Here's how the part is built. I have some questions about the finished solid (model axes, mm). A direction names the side the tool comes from. Coordinates: 2 decimals unless noted, no trailing zeros. Loops run counter-clockwise (first coordinate to the right, second up) from the corner with the lowest first, then second, coordinate; pieces in that order, holes last. Notation, with made-up numbers: (74.25, 62) -> (107.25, 62) arc R29 ccw to (107.25, 86) -> close; hole circle Ø1 at (-38.5, 3.25). An arc over 180 degrees is marked (long way). Answer as a JSON object with one key per item and string values. Group by question number.
Q1. I want a section at B-B on y = -5. Write out the boundary of the cut face in (x, z).
Q2. I need wall thicknesses on line 1 (Z direction, x = -19, y = -0.5); line 2 (X direction, y = -6.5, z = -31); line 3 (Z direction, x = -10, y = -2.5). Which ranges of each line are inside material? Lowest first, please.
Q3. Thinking about a two-plate mould opening in Z: for faces 1 (the flat face through (6, -3, -34.366)), 2 (the flat face through (0, -4, 29.286)), 3 (the flat face through (15, -7.62, -31)), which applies, released by +Z, released by -Z, zero draft, split by the parting line, or undercut?
Q4. I want a section at A-A on z = 6.5. Write out the boundary of the cut face in (x, y), then the cut area to 3 significant figures.
Q5. I want a section at D-D on x = 18. Write out the boundary of the cut face in (y, z), then the cut area to 3 significant figures.
Q6. I'm going to push flat-ended pins straight in: pin 1 (3 mm diameter, centred on x = -17.5, z = -5.5, fed in from -Y); pin 2 (3 mm diameter, centred on x = 2.5, z = 22.5, fed in from -Y); pin 3 (2.5 mm diameter, centred on x = -12, z = -32, fed in from -Y). Where does each tip first touch, or does it pass through?
Q7. On a 3-axis mill with a long thin cutter (end or side, diameter ignored), from which of +Z, -Z, +X, -X, +Y, -Y can I reach the whole of each face in a straight line? I mean faces 4 (the flat face through (-26.988, -2, -2)), 5 (the flat face through (-22, -2.54, -32)), 6 (the flat face through (18, -1.27, 0)). Say none if no direction works.
Q8. I want a section at C-C on z = -15.5. Write out the boundary of the cut face in (x, y).
Autodesk Inventor part; units mm, degrees
ref_plane "YZ Plane" through (0, 0, 0) normal (1, 0, 0) x (0, 1, 0)
ref_plane "XZ Plane" through (0, 0, 0) normal (0, 1, 0) x (-1, 0, 0)
ref_plane "XY Plane" through (0, 0, 0) normal (0, 0, 1) x (1, 0, 0)
sketch "Top Plate" plane through (0, 0, 0) normal (0, 1, 0) x (-1, 0, 0)
  line L0 (-26.9875, 30.5562) -> (26.9875, 30.5562)
  line L1 (26.9875, 30.5562) -> (26.9875, -30.5562)
  line L2 (26.9875, -30.5562) -> (-26.9875, -30.5562)
  line L3 (-26.9875, -30.5562) -> (-26.9875, 30.5562)
  line L4 (-26.9875, 30.5562) -> (26.9875, -30.5562) construction
  line L5 (26.9875, 30.5562) -> (-26.9875, -30.5562) construction
  line L6 (19.3675, 20.3962) -> (-14.9225, 20.3962)
  line L7 (-14.9225, 20.3962) -> (-14.9225, -24.0538)
  line L8 (-14.9225, -24.0538) -> (19.3675, -24.0538)
  line L9 (19.3675, -24.0538) -> (19.3675, 20.3962)
  line L10 (18.9103, 30.5562) -> (18.2753, 30.5562)
  line L11 (12.3825, 28.0162) -> (13.0175, 28.0162)
  line L12 (13.0175, 28.0162) -> (13.0175, 30.5562)
  line L13 (13.0175, 30.5562) -> (12.3825, 30.5562)
  line L14 (12.3825, 30.5562) -> (12.3825, 28.0162)
  line L15 (26.9875, -30.5562) -> (-26.9875, -30.5562)
  line L16 (-26.9875, -30.5562) -> (-26.9875, -34.3662)
  line L17 (-26.9875, -34.3662) -> (26.9875, -34.3662)
  line L18 (26.9875, -34.3662) -> (26.9875, -30.5562)
  point P0 (0, 0)
  dimension "d0" = 53.975
  dimension "d1" = 61.1124
  dimension "d7" = 44.45
  dimension "d8" = 34.29
  dimension "d9" = 7.62
  dimension "d10" = 10.16
  dimension "d48" = 0.635
  dimension "d49" = 6.35
  dimension "d50" = 2.54
  dimension "d77" = 3.81
extrude "Top Plate Ext" add sketch "Top Plate" against normal blind 7.62 contours L0 L14 L11 L12 L1 L2 L3 | L0 L12 L11 L14 | L9 L8 L7 L6
shell "Top Plate Shell" thickness 1.27 removed faces 1 at (8.9958, -7.62, 10.1854)
extrude "Display Cutout" cut sketch "Top Plate" against normal blind 1.27 contours L9 L8 L7 L6
sketch "Power Btn" plane through (26.9875, 0, 30.5562) normal (1, 0, 0) x (0, 0, -1)
  line L0 (59.8424, -7.62) -> (1.27, -7.62)
  line L1 (59.2074, -7.62) -> (34.4424, -7.62)
  line L2 (34.4424, -7.62) -> (34.4424, -2.54)
  line L3 (34.4424, -2.54) -> (59.2074, -2.54)
  line L4 (59.2074, -2.54) -> (59.2074, -7.62)
  line L5 (61.1124, 0) -> (61.1124, -7.62)
  line L6 (61.1124, 0) -> (0, 0)
  point P0 (30.5562, 0)
  dimension "d18" = 1.905
  dimension "d19" = 24.765
  dimension "d20" = 2.54
sketch "Dial/Vol" plane through (26.9875, 0, -30.5562) normal (0, 0, -1) x (-1, 0, 0)
  line L0 (53.975, -7.62) -> (0, -7.62)
  line L1 (52.705, -7.62) -> (46.355, -7.62)
  line L2 (46.355, -7.62) -> (46.355, -2.54)
  line L3 (46.355, -2.54) -> (52.705, -2.54)
  line L4 (52.705, -2.54) -> (52.705, -7.62)
  line L5 (53.975, 0) -> (0, 0)
  line L6 (52.705, -1.27) -> (52.705, -7.62)
  line L7 (1.27, -7.62) -> (52.705, -7.62)
  line L8 (44.323, -7.62) -> (25.273, -7.62)
  line L9 (25.273, -7.62) -> (25.273, -2.54)
  line L10 (25.273, -2.54) -> (44.323, -2.54)
  line L11 (44.323, -2.54) -> (44.323, -7.62)
  point P0 (26.9875, 0)
  dimension "d23" = 2.54
  dimension "d24" = 6.35
  dimension "d25" = 2.032
  dimension "d26" = 19.05
extrude "Power Cutout" cut sketch "Power Btn" against normal blind 1.27
extrude "Dial/Vol Cutout1" cut sketch "Dial/Vol" along normal blind 3.81 and the other way blind 1.27
sketch "SD Port" plane through (-26.9875, 0, -30.5562) normal (-1, 0, 0) x (0, 0, 1)
  line L0 (22.3774, -6.604) -> (46.5074, -6.604)
  line L1 (46.5074, -6.604) -> (46.5074, -2.794)
  line L2 (46.5074, -2.794) -> (22.3774, -2.794)
  line L3 (22.3774, -2.794) -> (22.3774, -6.604)
  line L4 (61.1124, 0) -> (0, 0)
  point P0 (30.5562, 0)
  point P1 (50.9524, 0)
  dimension "d31" = 2.794
  dimension "d32" = 3.81
  dimension "d33" = 24.13
  dimension "d34" = 4.445
extrude "SD Port Cutout" cut sketch "SD Port" against normal blind 1.27
sketch "Display Pins" plane through (-25.7175, -1.27, -29.2862) normal (0, -1, 0) x (1, 0, 0)
  line L0 (40.64, 50.9524) -> (6.35, 50.9524)
  line L1 (6.35, 50.9524) -> (6.35, 53.4924)
  line L2 (6.35, 53.4924) -> (40.64, 53.4924)
  line L3 (40.64, 53.4924) -> (40.64, 50.9524)
  line L4 (40.64, 49.6824) -> (40.64, 5.2324)
  line L5 (6.35, 5.2324) -> (6.35, 49.6824)
  point P0 (25.7175, 29.2862)
  dimension "d56" = 1.27
  dimension "d57" = 2.54
extrude "Display Pins Cutout" cut sketch "Display Pins" against normal blind 1.016
extrude "M3 Screw Ext" add sketch "Top Plate" against normal blind 7.62 contours L2 L18 L17 L16
extrude "Dial/Vol Cutout2" cut sketch "Dial/Vol" along normal blind 7.62
properties part number "lisa"
Result set:
{
 "1": {"outline": "(-26.99, -34.37) -> (-25.72, -34.37) -> (-25.72, -8.18) -> (-26.99, -8.18) -> close; (-26.99, 15.95) -> (-25.72, 15.95) -> (-25.72, 29.29) -> (25.72, 29.29) -> (25.72, -3.89) -> (26.99, -3.89) -> (26.99, 30.56) -> (-26.99, 30.56) -> close; (-19.37, -34.37) -> (-17.34, -34.37) -> (-17.34, -29.29) -> (-19.37, -29.29) -> close; (1.71, -34.37) -> (26.99, -34.37) -> (26.99, -28.65) -> (25.72, -28.65) -> (25.72, -29.29) -> (1.71, -29.29) -> close"},
 "2": {"line 1": "z = -34.37 to -24.05, 20.4 to 21.67, 24.21 to 30.56", "line 2": "x = -26.99 to -25.72, -19.37 to -17.34, 1.71 to 26.99", "line 3": "z = -34.37 to -29.29, 29.29 to 30.56"},
 "3": {"face 1": "released by -Z", "face 2": "undercut", "face 3": "zero draft"},
 "4": {"outline": "(-26.99, -7.62) -> (-25.72, -7.62) -> (-25.72, -6.6) -> (-26.99, -6.6) -> close; (-26.99, -2.79) -> (-25.72, -2.79) -> (-25.72, -1.27) -> (-19.37, -1.27) -> (-19.37, 0) -> (-26.99, 0) -> close; (14.92, -1.27) -> (25.72, -1.27) -> (25.72, -7.62) -> (26.99, -7.62) -> (26.99, 0) -> (14.92, 0) -> close", "area": "36.3 mm²"},
 "5": {"outline": "(-7.62, -34.37) -> (0, -34.37) -> (0, 30.56) -> (-7.62, 30.56) -> (-7.62, 29.29) -> (-1.27, 29.29) -> (-1.27, -29.29) -> (-7.62, -29.29) -> close", "area": "123 mm²"},
 "6": {"pin 1": "passes through", "pin 2": "stops at y = -1.27", "pin 3": "stops at y = -2.54"},
 "7": {"face 4": "+Z, -Z, -X, +Y, -Y", "face 5": "-Z, -Y", "face 6": "-Y"},
 "8": {"outline": "(-26.99, -7.62) -> (-25.72, -7.62) -> (-25.72, -1.27) -> (-19.37, -1.27) -> (-19.37, 0) -> (-26.99, 0) -> close; (14.92, -1.27) -> (25.72, -1.27) -> (25.72, -2.54) -> (26.99, -2.54) -> (26.99, 0) -> (14.92, 0) -> close"}
}
